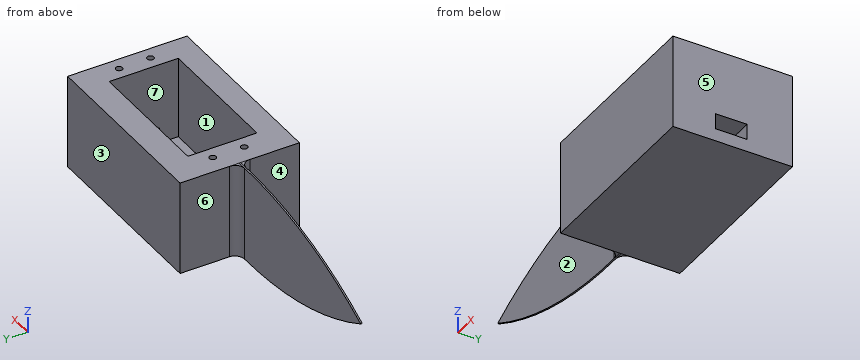
```python
from build123d import *

# Parameters (mm, degrees)
BOSS_EXTRUDE1_DEPTH  = 4
CUT_EXTRUDE1_DEPTH   = 3
SKETCH5_W            = 49
SKETCH5_H            = 16
BOSS_EXTRUDE2_DEPTH  = 4
BOSS_EXTRUDE15_DEPTH = 30
SKETCH20_R           = 2.4
CUT_EXTRUDE26_DEPTH  = 1
FILLET8_R            = 4
FILLET12_R           = 4
CUT_EXTRUDE_8_DEPTH  = 28
SKETCH_6_R           = 1.05
CUT_EXTRUDE_9_DEPTH  = 20
SKETCH_8_W           = 6
SKETCH_8_H           = 10
CUT_EXTRUDE_10_DEPTH = 8
BOSS_EXTRUDE14_DEPTH = 4
CUT_EXTRUDE27_DEPTH  = 19
BOSS_EXTRUDE16_DEPTH = 19.25
CUT_EXTRUDE28_DEPTH  = 18.75
FILLET13_R           = 3
FILLET14_R           = 3


with BuildPart() as part:
    # Sketch2 → Boss-Extrude1 (new body)
    with BuildSketch(Plane.XY):
        with BuildLine():
            Line((23.733047461, 11.63962887), (23.733047461, -4.36037113))
            Line((23.733047461, -4.36037113), (-21.266952539, -4.36037113))
            ThreePointArc((-21.266952539, -4.36037113), (-27.597931628, 3.63962887), (-21.266952539, 11.63962887))
            Line((-21.266952539, 11.63962887), (23.733047461, 11.63962887))
        make_face()
    extrude(amount=BOSS_EXTRUDE1_DEPTH)

    # Sketch1 → Cut-Extrude1 (cut)
    with BuildSketch(Plane.XY):
        with BuildLine():
            Line((-6.25004119, 8.63962887), (-20.04279291, 6.23962887))
            ThreePointArc((-20.04279291, 6.23962887), (-22.105421524, 3.63962887), (-20.04279291, 1.03962887))
            Line((-20.04279291, 1.03962887), (-6.25004119, -1.36037113))
            ThreePointArc((-6.25004119, -1.36037113), (-2.105421524, -2.86037113), (2.039198142, -1.36037113))
            Line((2.039198142, -1.36037113), (15.831949862, 1.03962887))
            ThreePointArc((15.831949862, 1.03962887), (17.894578476, 3.63962887), (15.831949862, 6.23962887))
            Line((15.831949862, 6.23962887), (2.039198142, 8.63962887))
            ThreePointArc((2.039198142, 8.63962887), (-2.105421524, 10.13962887), (-6.25004119, 8.63962887))
        make_face()
    extrude(amount=CUT_EXTRUDE1_DEPTH, mode=Mode.SUBTRACT)

    # Sketch5 → Boss-Extrude2 (add)
    with BuildSketch(Plane(origin=(23.733047461, 0, 0), x_dir=(0, 0, -1), z_dir=(1, 0, 0))):
        with Locations((20.5, 3.63962887)):
            Rectangle(SKETCH5_W, SKETCH5_H)
    extrude(amount=BOSS_EXTRUDE2_DEPTH)

    # Sketch6 → Boss-Extrude15 (add)
    with BuildSketch(Plane(origin=(0, 0, -45), x_dir=(-1, 0, 0), z_dir=(0, 0, -1))):
        Polygon((-30.946192459, -15.36037113), (-83.733047461, -15.36037113), (-83.733047461, 22.63962887), (-23.733047461, 22.63962887), (-23.733047461, -15.36037113), align=None)
    extrude(amount=-BOSS_EXTRUDE15_DEPTH)

    # Sketch20 → Cut-Extrude26 (cut)
    with BuildSketch(Plane(origin=(0, 0, 3), x_dir=(-1, 0, 0), z_dir=(0, 0, -1))):
        with Locations((2.105421524, 3.63962887)):
            Circle(SKETCH20_R)
    extrude(amount=-CUT_EXTRUDE26_DEPTH, mode=Mode.SUBTRACT)

    # Fillet8
    fillet8_edges = [part.edges().sort_by_distance(p)[0] for p in [
        (23.733047461, 3.63962887, 0),
    ]]
    fillet(fillet8_edges, radius=FILLET8_R)

    # Fillet12
    fillet12_edges = [part.edges().sort_by_distance(p)[0] for p in [
        (27.733047461, 3.63962887, 4),
    ]]
    fillet(fillet12_edges, radius=FILLET12_R)

    # 草圖5 → 除料-伸長8 (cut)
    with BuildSketch(Plane.XY.offset(-15)):
        Polygon((75.733047461, -7.806095257), (75.733047461, 14.193904743), (33.733047461, 14.193904743), (33.733047461, 3.193904743), (33.733047461, -7.806095257), align=None)
    extrude(amount=-CUT_EXTRUDE_8_DEPTH, mode=Mode.SUBTRACT)

    # 草圖6 → 除料-伸長9 (cut)
    with BuildSketch(Plane.XY.offset(-15)):
        with Locations((29.733047461, 8.63962887)):
            Circle(SKETCH_6_R)
        with Locations((29.733047461, -1.36037113)):
            Circle(SKETCH_6_R)
        with Locations((79.733047461, 8.63962887)):
            Circle(SKETCH_6_R)
        with Locations((79.733047461, -1.36037113)):
            Circle(SKETCH_6_R)
    extrude(amount=-CUT_EXTRUDE_9_DEPTH, mode=Mode.SUBTRACT)

    # 草圖8 → 除料-伸長10 (cut)
    with BuildSketch(Plane(origin=(83.733047461, 0, 0), x_dir=(0, 0, -1), z_dir=(1, 0, 0))):
        with Locations((39, 3.238584995)):
            Rectangle(SKETCH_8_W, SKETCH_8_H)
    extrude(amount=-CUT_EXTRUDE_10_DEPTH, mode=Mode.SUBTRACT)

    # Sketch6<2> → Boss-Extrude14 (add)
    with BuildSketch(Plane(origin=(0, 0, -45), x_dir=(-1, 0, 0), z_dir=(0, 0, -1))):
        Polygon((-30.946192459, -15.36037113), (-83.733047461, -15.36037113), (-83.733047461, 22.63962887), (-23.733047461, 22.63962887), (-23.733047461, -15.36037113), align=None)
    extrude(amount=-BOSS_EXTRUDE14_DEPTH)

    # Sketch21 → Cut-Extrude27 (cut)
    with BuildSketch(Plane.XY.offset(4)):
        Polygon((-21.266952539, 11.63962887), (23.733047461, 11.63962887), (27.733047461, 11.63962887), (27.733047461, -4.36037113), (-21.266952539, -4.36037113), (-27.597931628, -4.36037113), (-27.597931628, 3.63962887), (-27.597931628, 11.63962887), align=None)
    extrude(amount=-CUT_EXTRUDE27_DEPTH, mode=Mode.SUBTRACT)

    # Sketch26 → Boss-Extrude16 (add)
    with BuildSketch(Plane(origin=(0, 22.63962887, 0), x_dir=(1, 0, 0), z_dir=(0, 1, 0))):
        with BuildLine():
            Line((23.733047461, 45), (23.733047461, 15))
            ThreePointArc((23.733047461, 15), (-9.769414537, 18.155998007), (-41.266952539, 30))
            ThreePointArc((-41.266952539, 30), (-9.769414537, 41.844001993), (23.733047461, 45))
        make_face()
    extrude(amount=-BOSS_EXTRUDE16_DEPTH)

    # Sketch26<2> → Cut-Extrude28 (cut)
    with BuildSketch(Plane(origin=(0, 22.63962887, 0), x_dir=(1, 0, 0), z_dir=(0, 1, 0))):
        with BuildLine():
            Line((23.733047461, 45), (23.733047461, 15))
            ThreePointArc((23.733047461, 15), (-9.769414537, 18.155998007), (-41.266952539, 30))
            ThreePointArc((-41.266952539, 30), (-9.769414537, 41.844001993), (23.733047461, 45))
        make_face()
    extrude(amount=-CUT_EXTRUDE28_DEPTH, mode=Mode.SUBTRACT)

    # Fillet13
    # the kernel refuses this fillet: 3 mm, written as the material it adds along each edge
    with BuildSketch(Plane(origin=(23.733047461, 3.38962887, -52.5), x_dir=(0, -1, 0), z_dir=(0, 0, 1))) as fillet13_piece_1_section:
        with BuildLine():
            CenterArc((FILLET13_R, -FILLET13_R), FILLET13_R, 90, 90)
            Line((0, -FILLET13_R), (0, 0))
            Line((0, 0), (FILLET13_R, 0))
        make_face()
    fillet13_piece_1 = extrude(amount=37.5, mode=Mode.PRIVATE)
    fillet13_piece_1 = split(fillet13_piece_1, bisect_by=Plane(origin=(22.499991294, 3.049704753, -45), z_dir=(0, 0, -1)), keep=Keep.TOP, mode=Mode.PRIVATE)
    fillet13_piece_1 = fillet13_piece_1 & Plane(origin=(18.787742814, 3.049704753, 81.90367986), x_dir=(-0.472871616946814, 0, -0.8811313374781911), z_dir=(0, 1, 0)) * Cylinder(127, 87, mode=Mode.PRIVATE)
    add(fillet13_piece_1)
    with BuildSketch(Plane(origin=(23.733047461, 3.38962887, -45), x_dir=(0, -1, 0), z_dir=(0, 0, 1))) as fillet13_piece_2:
        with BuildLine():
            CenterArc((FILLET13_R, -FILLET13_R), FILLET13_R, 90, 90)
            Line((0, -FILLET13_R), (0, 0))
            Line((0, 0), (FILLET13_R, 0))
        make_face()
    extrude(amount=30)
    with BuildSketch(Plane(origin=(23.733047461, 3.38962887, -45), x_dir=(0, -1, 0), z_dir=(0, 0, 1))) as fillet13_piece_3_section:
        with BuildLine():
            CenterArc((FILLET13_R, -FILLET13_R), FILLET13_R, 90, 90)
            Line((0, -FILLET13_R), (0, 0))
            Line((0, 0), (FILLET13_R, 0))
        make_face()
    fillet13_piece_3 = extrude(amount=37.5, mode=Mode.PRIVATE)
    fillet13_piece_3 = split(fillet13_piece_3, bisect_by=Plane(origin=(22.499977065, 3.049704014, -15), z_dir=(0, 0, 1)), keep=Keep.TOP, mode=Mode.PRIVATE)
    fillet13_piece_3 = fillet13_piece_3 & Plane(origin=(18.787742814, 3.049704014, -141.90367986), x_dir=(0.03893940667523239, 0, 0.9992415736986632), z_dir=(0, 1, 0)) * Cylinder(127, 87, mode=Mode.PRIVATE)
    add(fillet13_piece_3)

    # Fillet14
    # the kernel refuses this fillet: 3 mm, written as the material it adds along each edge
    with BuildSketch(Plane(origin=(23.733047461, 3.88962887, -52.5), x_dir=(-1, 0, 0), z_dir=(0, 0, 1))) as fillet14_piece_1_section:
        with BuildLine():
            CenterArc((FILLET14_R, -FILLET14_R), FILLET14_R, 90, 90)
            Line((0, -FILLET14_R), (0, 0))
            Line((0, 0), (FILLET14_R, 0))
        make_face()
    fillet14_piece_1 = extrude(amount=37.5, mode=Mode.PRIVATE)
    fillet14_piece_1 = fillet14_piece_1 & Plane(origin=(18.787742814, 4.229564141, 81.90367986), x_dir=(-0.472871616947038, 0, -0.8811313374780708), z_dir=(0, 1, 0)) * Cylinder(127, 87, mode=Mode.PRIVATE)
    fillet14_piece_1 = split(fillet14_piece_1, bisect_by=Plane(origin=(22.499997124, 4.229564141, -45), z_dir=(0, 0, -1)), keep=Keep.TOP, mode=Mode.PRIVATE)
    add(fillet14_piece_1)
    with BuildSketch(Plane(origin=(23.733047461, 3.88962887, -45), x_dir=(-1, 0, 0), z_dir=(0, 0, 1))) as fillet14_piece_2:
        with BuildLine():
            CenterArc((FILLET14_R, -FILLET14_R), FILLET14_R, 90, 90)
            Line((0, -FILLET14_R), (0, 0))
            Line((0, 0), (FILLET14_R, 0))
        make_face()
    extrude(amount=30)
    with BuildSketch(Plane(origin=(23.733047461, 3.88962887, -45), x_dir=(-1, 0, 0), z_dir=(0, 0, 1))) as fillet14_piece_3_section:
        with BuildLine():
            CenterArc((FILLET14_R, -FILLET14_R), FILLET14_R, 90, 90)
            Line((0, -FILLET14_R), (0, 0))
            Line((0, 0), (FILLET14_R, 0))
        make_face()
    fillet14_piece_3 = extrude(amount=37.5, mode=Mode.PRIVATE)
    fillet14_piece_3 = fillet14_piece_3 & Plane(origin=(18.787742814, 4.229551156, -141.90367986), x_dir=(0.03893940667498725, 0, 0.9992415736986727), z_dir=(0, 1, 0)) * Cylinder(127, 87, mode=Mode.PRIVATE)
    fillet14_piece_3 = split(fillet14_piece_3, bisect_by=Plane(origin=(22.499980416, 4.229551156, -15), z_dir=(0, 0, 1)), keep=Keep.TOP, mode=Mode.PRIVATE)
    add(fillet14_piece_3)


solid = part.part
```
Can you work these out from the model? Positions are in its coordinate system, mm. Face numbers are marked on the shaded views. A direction names the side the tool comes from. Give positions to 0.01 mm unless a question says otherwise; leave off trailing zeros. Loops run counter-clockwise (first coordinate to the right, second up) from the corner with the lowest first, then second, coordinate; pieces in that order, holes last. Notation, with made-up numbers: M 45,-20 L 57,-20 A21 cw 57,12 Z; hole C 21,45 d9. An arc over 180 degrees is marked long. One line per question, with ' | ' between items. Start each with the question number.
Q1. If I drill on line 1 (X direction, y = -6.5, z = -33.5); line 2 (Y direction, x = 66, z = -26.5); line 3 (X direction, y = 21, z = -21), over which ranges is the centre line in solid material (lowest first)? Write a range as from..to.
Q2. For the marked faces 5, 6 and 7, which set-ups out of +Z, -Z, +X, -X, +Y, -Y let a thin tool reach every point of the face, with its end or its side?
Q3. If we section it at B-B (z = -22.5): Please give me the cut outline in (x, y), plus the area to 3 significant figures.
Q4. For pin 1 Ø1.5 at (x, y) = (62.5, 18.5) entering from -Z; pin 2 Ø8 at (y, z) = (17, -21.5) entering from -X; pin 3 Ø9 at (x, z) = (-19, -28.5) entering from +Y, each with a flat end and sliding along its axis, tell me the tip position at first contact or that it passes through.
Q5. If we mould it in two halves opening along Y, with no side actions, what happens to the marked faces 1, 2, 3 and 4? For each: +Y half, -Y half, draft (parallel to the pull), parting line (faces both ways), or undercut.
Q6. If we section it at D-D (z = -32.5): Please give me the cut outline in (x, y), plus the area to 3 significant figures.
Q7. If we section it at A-A (x = 60.5): Please give me the cut outline in (y, z), plus the area to 3 significant figures.
Q8. If we section it at C-C (y = 11): Please give me the cut outline in (x, z), plus the area to 3 significant figures.
Computed:
1) line 1: x = 23.73..33.73, 75.73..83.73 | line 2: y = -15.36..-7.81, 14.19..22.64 | line 3: x = 23.73..83.73
2) face 5: +Z, -Z, +X, +Y, -Y | face 6: +Z, -Z, -X, +Y | face 7: +Z
3) outline: M -24.48,3.39 L 20.73,3.39 A3 cw 23.73,0.39 L 23.73,-15.36 L 83.73,-15.36 L 83.73,22.64 L 23.73,22.64 L 23.73,6.89 A3 cw 20.73,3.89 L -24.48,3.89 Z; hole C 29.73,-1.36 d2.1; hole C 29.73,8.64 d2.1; hole M 33.73,-7.81 L 75.73,-7.81 L 75.73,14.19 L 33.73,14.19 Z; hole C 79.73,-1.36 d2.1; hole C 79.73,8.64 d2.1 | area: 1,370 mm²
4) pin 1: stops at z = -45 | pin 2: stops at x = 23.73 | pin 3: stops at y = 3.89
5) face 1: undercut | face 2: -Y half | face 3: +Y half | face 4: draft
6) outline: M -36.36,3.39 L 20.73,3.39 A3 cw 23.73,0.39 L 23.73,-15.36 L 83.73,-15.36 L 83.73,22.64 L 23.73,22.64 L 23.73,6.89 A3 cw 20.73,3.89 L -36.36,3.89 Z; hole C 29.73,-1.36 d2.1; hole C 29.73,8.64 d2.1; hole M 33.73,-7.81 L 75.73,-7.81 L 75.73,14.19 L 33.73,14.19 Z; hole C 79.73,-1.36 d2.1; hole C 79.73,8.64 d2.1 | area: 1,380 mm²
7) outline: M -15.36,-45 L 22.64,-45 L 22.64,-15 L 14.19,-15 L 14.19,-41 L -7.81,-41 L -7.81,-15 L -15.36,-15 Z | area: 568 mm²
8) outline: M 23.73,-45 L 83.73,-45 L 83.73,-15 L 75.73,-15 L 75.73,-41 L 33.73,-41 L 33.73,-15 L 23.73,-15 Z | area: 708 mm²
